Autodesk Inventor part; units mm, degrees
ref_plane "YZ Plane" through (0, 0, 0) normal (1, 0, 0) x (0, 1, 0)
ref_plane "XZ Plane" through (0, 0, 0) normal (0, 1, 0) x (-1, 0, 0)
ref_plane "XY Plane" through (0, 0, 0) normal (0, 0, 1) x (1, 0, 0)
sketch "Sketch1" plane through (0, 0, 0) normal (0, 0, 1) x (1, 0, 0)
  circle A0 centre (45.5, -15.3826) radius 3
  circle A1 centre (-45.5, -15.3826) radius 3
  line L0 (44.6636, 0.7689) -> (35.6636, 0.7689)
  line L1 (33.6636, 2.7689) -> (33.6636, 5.2689)
  line L2 (46.6636, 5.2689) -> (46.6636, 2.7689)
  line L3 (29.9455, -2.1666) -> (-2.0545, -2.1666)
  line L4 (-4.0545, -0.1666) -> (-4.0545, 2.8334)
  line L5 (31.9455, 2.8334) -> (31.9455, -0.1666)
  circle A2 centre (89.024, -15.4039) radius 1.5
  circle A3 centre (65.024, -15.4039) radius 1.5
  circle A4 centre (89.024, 8.5961) radius 1.5
  circle A5 centre (65.024, 8.5961) radius 1.5
  arc A6 (67.8322, 7.6809) -> (67.8322, -14.4886) centre (77.024, -3.4039) ccw
  line L6 (69.3366, 7.4111) -> (71.8641, 3.0334)
  arc A7 (71.8641, 3.0334) -> (71.8641, -9.8411) centre (77.024, -3.4039) ccw
  line L7 (71.8641, -9.8411) -> (69.3366, -14.2188)
  arc A8 (67.8322, -14.4886) -> (69.3366, -14.2188) centre (68.4705, -13.7188) ccw
  arc A9 (69.3366, 7.4111) -> (67.8322, 7.6809) centre (68.4705, 6.9111) ccw
  arc A10 (91.2195, -0.986) -> (72.0202, 10.0988) centre (77.024, -3.4039) ccw
  arc A11 (72.0202, 10.0988) -> (71.5016, 8.6611) centre (72.3677, 9.1611) ccw
  line L8 (74.0291, 4.2834) -> (71.5016, 8.6611)
  arc A12 (85.1787, -2.1539) -> (74.0291, 4.2834) centre (77.024, -3.4039) ccw
  line L9 (90.2337, -2.1539) -> (85.1787, -2.1539)
  arc A13 (90.2337, -2.1539) -> (91.2195, -0.986) centre (90.2337, -1.1539) ccw
  line L10 (85.1787, -4.6539) -> (90.2337, -4.6539)
  arc A14 (91.2195, -5.8218) -> (90.2337, -4.6539) centre (90.2337, -5.6539) ccw
  arc A15 (72.0202, -16.9065) -> (91.2195, -5.8218) centre (77.024, -3.4039) ccw
  arc A16 (71.5016, -15.4688) -> (72.0202, -16.9065) centre (72.3677, -15.9688) ccw
  line L11 (71.5016, -15.4688) -> (74.0291, -11.0911)
  arc A17 (74.0291, -11.0911) -> (85.1787, -4.6539) centre (77.024, -3.4039) ccw
  circle A18 centre (-64.8953, -15.374) radius 1.5
  circle A19 centre (-88.8953, -15.374) radius 1.5
  circle A20 centre (-88.8953, 8.626) radius 1.5
  circle A21 centre (-64.8953, 8.626) radius 1.5
  arc A22 (-62.6997, -0.956) -> (-81.8991, 10.1287) centre (-76.8953, -3.374) ccw
  arc A23 (-81.8991, 10.1287) -> (-82.4176, 8.691) centre (-81.5516, 9.191) ccw
  line L12 (-79.8901, 4.3133) -> (-82.4176, 8.691)
  line L13 (-84.5827, 7.441) -> (-82.0552, 3.0633)
  arc A24 (-84.5827, 7.441) -> (-86.087, 7.7108) centre (-85.4487, 6.941) ccw
  arc A25 (-86.087, 7.7108) -> (-86.087, -14.4587) centre (-76.8953, -3.374) ccw
  arc A26 (-82.0552, 3.0633) -> (-82.0552, -9.8112) centre (-76.8953, -3.374) ccw
  arc A27 (-68.7405, -2.124) -> (-79.8901, 4.3133) centre (-76.8953, -3.374) ccw
  line L14 (-63.6855, -2.124) -> (-68.7405, -2.124)
  arc A28 (-63.6855, -2.124) -> (-62.6997, -0.956) centre (-63.6855, -1.124) ccw
  line L15 (-68.7405, -4.624) -> (-63.6855, -4.624)
  arc A29 (-62.6997, -5.7919) -> (-63.6855, -4.624) centre (-63.6855, -5.624) ccw
  arc A30 (-81.8991, -16.8766) -> (-62.6997, -5.7919) centre (-76.8953, -3.374) ccw
  arc A31 (-79.8901, -11.0612) -> (-68.7405, -4.624) centre (-76.8953, -3.374) ccw
  line L16 (-82.4176, -15.4389) -> (-79.8901, -11.0612)
  arc A32 (-82.4176, -15.4389) -> (-81.8991, -16.8766) centre (-81.5516, -15.9389) ccw
  line L17 (-82.0552, -9.8112) -> (-84.5827, -14.1889)
  arc A33 (-86.087, -14.4587) -> (-84.5827, -14.1889) centre (-85.4487, -13.6889) ccw
  line L18 (-2.0545, 4.8334) -> (29.9455, 4.8334)
  line L19 (35.6636, 7.2689) -> (44.6636, 7.2689)
  arc A34 (-4.0545, -0.1666) -> (-2.0545, -2.1666) centre (-2.0545, -0.1666) ccw
  arc A35 (-2.0545, 4.8334) -> (-4.0545, 2.8334) centre (-2.0545, 2.8334) ccw
  arc A36 (31.9455, 2.8334) -> (29.9455, 4.8334) centre (29.9455, 2.8334) ccw
  arc A37 (29.9455, -2.1666) -> (31.9455, -0.1666) centre (29.9455, -0.1666) ccw
  arc A38 (33.6636, 2.7689) -> (35.6636, 0.7689) centre (35.6636, 2.7689) ccw
  arc A39 (35.6636, 7.2689) -> (33.6636, 5.2689) centre (35.6636, 5.2689) ccw
  arc A40 (46.6636, 5.2689) -> (44.6636, 7.2689) centre (44.6636, 5.2689) ccw
  arc A41 (44.6636, 0.7689) -> (46.6636, 2.7689) centre (44.6636, 2.7689) ccw
  line L20 (-87.4504, 24.6174) -> (-57.4504, 24.6174)
  line L21 (-87.4504, 19.6174) -> (-87.4504, 24.6174)
  line L22 (-87.4504, 19.6174) -> (-57.4504, 19.6174)
  line L23 (-57.4504, 19.6174) -> (-57.4504, 24.6174)
  line L24 (-27.4504, 19.6174) -> (27.5496, 19.6174)
  line L25 (27.5496, 19.6174) -> (27.5496, 24.6174)
  line L26 (-27.4504, 24.6174) -> (27.5496, 24.6174)
  line L27 (-27.4504, 19.6174) -> (-27.4504, 24.6174)
  line L28 (57.5496, 19.6174) -> (87.5496, 19.6174)
  line L29 (87.5496, 19.6174) -> (87.5496, 24.6174)
  line L30 (57.5496, 24.6174) -> (87.5496, 24.6174)
  line L31 (57.5496, 19.6174) -> (57.5496, 24.6174)
  line L32 (-98.9504, -25.3833) -> (-98.9504, -33.3826)
  line L33 (99.0496, -33.3826) -> (-98.9504, -33.3826)
  line L34 (-98.9504, 24.6174) -> (-93.9504, 24.6174)
  line L35 (-93.9504, 24.6174) -> (-93.9504, 9.6159)
  line L36 (-98.9504, 9.6159) -> (-93.9504, 9.6159)
  line L37 (-98.9504, 9.6159) -> (-98.9504, -10.3841)
  line L38 (-98.9504, -10.3841) -> (-93.9504, -10.3841)
  line L39 (-93.9504, -10.3841) -> (-93.9504, -25.3833)
  line L40 (-98.9504, -25.3833) -> (-93.9504, -25.3833)
  line L41 (99.0496, -25.3833) -> (99.0496, -33.3833)
  line L42 (94.0496, -25.3833) -> (99.0496, -25.3833)
  line L43 (94.0496, -10.3841) -> (94.0496, -25.3833)
  line L44 (94.0496, -10.3841) -> (99.0496, -10.3841)
  line L45 (99.0496, 9.6159) -> (99.0496, -10.3841)
  line L46 (94.0496, 9.6159) -> (99.0496, 9.6159)
  line L47 (94.0496, 24.6174) -> (94.0496, 9.6159)
  line L48 (94.0496, 24.6174) -> (99.0496, 24.6174)
  line L49 (-98.9504, 24.6174) -> (-98.9504, 32.6174)
  line L50 (-98.9504, 32.6174) -> (99.0496, 32.6174)
  line L51 (99.0496, 32.6174) -> (99.0496, 24.6174)
  line L52 (-22.6436, -2.2792) -> (-22.6436, -8.2792)
  line L53 (-35.6436, -0.2792) -> (-24.6436, -0.2792)
  line L54 (-24.6436, -10.2792) -> (-35.6436, -10.2792)
  line L55 (-37.6436, -8.2792) -> (-37.6436, -2.2792)
  arc A42 (-35.6436, -0.2792) -> (-37.6436, -2.2792) centre (-35.6436, -2.2792) ccw
  arc A43 (-22.6436, -2.2792) -> (-24.6436, -0.2792) centre (-24.6436, -2.2792) ccw
  arc A44 (-24.6436, -10.2792) -> (-22.6436, -8.2792) centre (-24.6436, -8.2792) ccw
  arc A45 (-37.6436, -8.2792) -> (-35.6436, -10.2792) centre (-35.6436, -8.2792) ccw
  line L56 (-5.5869, 3.8805) -> (-5.5869, -1.877)
  line L57 (-7.5869, -3.877) -> (-13.5192, -3.877)
  line L58 (-15.5192, -1.877) -> (-15.5192, 3.8805)
  line L59 (-13.5192, 5.8805) -> (-7.5869, 5.8805)
  arc A46 (-13.5192, 5.8805) -> (-15.5192, 3.8805) centre (-13.5192, 3.8805) ccw
  arc A47 (-15.5192, -1.877) -> (-13.5192, -3.877) centre (-13.5192, -1.877) ccw
  arc A48 (-5.5869, 3.8805) -> (-7.5869, 5.8805) centre (-7.5869, 3.8805) ccw
  arc A49 (-7.5869, -3.877) -> (-5.5869, -1.877) centre (-7.5869, -1.877) ccw
  point P0 (-90.9348, -30.6649)
  point P1 (27.5, 24.6174)
  point P2 (0, 0)
  point P3 (-22.6436, -0.2792)
  point P4 (-22.6436, -10.2792)
  point P5 (-37.6436, -0.2792)
  point P6 (-37.6436, -10.2792)
  point P7 (-2.0545, 2.8334)
  dimension "d22" = 91
  dimension "d27" = 7
  dimension "d28" = 36
  dimension "d29" = 13
  dimension "d30" = 6.5
  dimension "d35" = 18
  dimension "d36" = 18
  dimension "d37" = 66
  dimension "d38" = 45.5
  dimension "d39" = 6
  dimension "d40" = 6
  dimension "d41" = 198
extrude "Extrusion1" add sketch "Sketch1" along normal blind 5
sketch "Sketch2" plane through (0, 0, 5) normal (0, 0, 1) x (1, 0, 0)
  line L0 (-44.5, 11.026) -> (44.5, 11.026)
  line L1 (48.5, 7.026) -> (48.5, -6.974)
  line L2 (44.5, -10.974) -> (-44.5, -10.974)
  line L3 (-48.5, -6.974) -> (-48.5, 7.026)
  arc A0 (-44.5, 11.026) -> (-48.5, 7.026) centre (-44.5, 7.026) ccw
  arc A1 (48.5, 7.026) -> (44.5, 11.026) centre (44.5, 7.026) ccw
  arc A2 (44.5, -10.974) -> (48.5, -6.974) centre (44.5, -6.974) ccw
  arc A3 (-48.5, -6.974) -> (-44.5, -10.974) centre (-44.5, -6.974) ccw
  line L4 (99.0496, -10.3841) -> (99.0496, 9.6159)
  line L5 (-98.9504, -33.3826) -> (99.0496, -33.3826)
  circle A4 centre (-45.5, -15.3826) radius 3
  circle A5 centre (45.5, -15.3826) radius 3
  arc A6 (-62.6997, -0.956) -> (-81.8991, 10.1287) centre (-76.8953, -3.374) ccw
  point P0 (0, 0)
  point P1 (-76.8953, -3.374)
  dimension "d48" = 4
  dimension "d58" = 97
  dimension "d59" = 22
  dimension "d60" = 50.5496
  dimension "d61" = 22.4087
extrude "Extrusion2" cut sketch "Sketch2" against normal up to next contours L0 A1 L1 A2 L2 A3 L3 A0
sketch "Sketch3" plane through (0, 0, 5) normal (0, 0, 1) x (1, 0, 0)
  line L0 (-92.421, 12.1859) -> (-62.2986, 12.1859)
  line L1 (-62.2986, 12.1859) -> (-62.2986, -19.0319)
  line L2 (-62.2986, -19.0319) -> (-92.421, -19.0319)
  line L3 (-92.421, -19.0319) -> (-92.421, 12.1859)
  line L4 (-92.421, 12.1859) -> (-62.2986, -19.0319) construction
  line L5 (-62.2986, 12.1859) -> (-92.421, -19.0319) construction
  line L6 (62.2986, 11.0377) -> (92.6949, 11.0377)
  line L7 (92.6949, 11.0377) -> (92.6949, -17.8837)
  line L8 (92.6949, -17.8837) -> (62.2986, -17.8837)
  line L9 (62.2986, -17.8837) -> (62.2986, 11.0377)
  line L10 (62.2986, 11.0377) -> (92.6949, -17.8837) construction
  line L11 (92.6949, 11.0377) -> (62.2986, -17.8837) construction
  point P0 (0, 0)
  point P1 (-77.3598, -3.423)
  point P2 (77.4968, -3.423)
extrude "Extrusion3" add sketch "Sketch3" against normal blind 10
properties part number "case bottom back" material "Titanium"
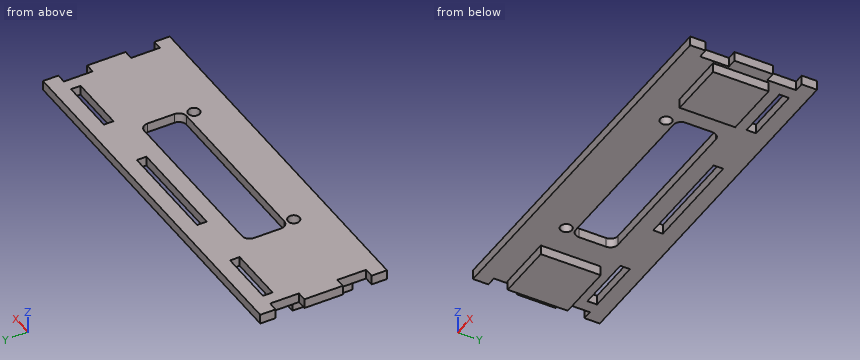
The model under review builds one solid part; all positions refer to its coordinate system, in mm. Round coordinates to 2 decimals unless told otherwise and drop trailing zeros. Order: outer loops, then holes, each group sorted by start corner. A loop starts at its lowest first (then second) coordinate and runs counter-clockwise, first axis right, second up. Notation, with made-up numbers: (-28.5, 17) -> (-23.5, 17) arc R29 ccw to (-23.5, 43) -> close; hole circle Ø6 at (84, -36.5). An arc over 180 degrees is marked (long way). Use a Markdown table: item, result.
Q1. We need section C-C on x = -60. Write out the cut boundary in (y, z), then the cut area to 3 significant figures.
Values:
| item | result |
|---|---|
| outline | (-33.38, 0) -> (19.62, 0) -> (19.62, 5) -> (-33.38, 5) -> close; (24.62, 0) -> (32.62, 0) -> (32.62, 5) -> (24.62, 5) -> close |
| area | 305 mm^2 |
Q2. For line 1 (Y direction, x = -59.5, z = 3); line 2 (X direction, y = 2, z = 0.75); line 3 (Y direction, x = -25.5, z = 1.5), list the stretches that pass through material, from the lowest coordinate up.
Values:
| item | result |
|---|---|
| line 1 | y = -33.38 to 19.62, 24.62 to 32.62 |
| line 2 | x = -98.95 to -48.5, 48.5 to 99.05 |
| line 3 | y = -33.38 to -10.97, 11.03 to 19.62, 24.62 to 32.62 |
Q3. We need section D-D on y = -21. Write out the cut boundary in (x, z).
Values:
| item | result |
|---|---|
| outline | (-93.95, 0) -> (94.05, 0) -> (94.05, 5) -> (-93.95, 5) -> close |
Q4. We need section A-A on x = -21. Write out the cut boundary in (y, z), then the cut area to 3 significant figures.
Values:
| item | result |
|---|---|
| outline | (-33.38, 0) -> (-10.97, 0) -> (-10.97, 5) -> (-33.38, 5) -> close; (11.03, 0) -> (19.62, 0) -> (19.62, 5) -> (11.03, 5) -> close; (24.62, 0) -> (32.62, 0) -> (32.62, 5) -> (24.62, 5) -> close |
| area | 195 mm^2 |
Q5. Clearance check with flat-ended pins moving along their axes: P1, Ø6, axis at x = -22, z = -4, coming from the +Y side; P2, Ø2.5, axis at y = -6, z = -2, coming from the +X side; P3, Ø1, axis at y = -6.5, z = -3, coming from the -X side; P4, Ø1.5, axis at y = 23, z = 2.5, coming from the -X side. State where each tip first meets the part, or that it passes through.
Values:
| item | result |
|---|---|
| P1 | passes through |
| P2 | stops at x = 92.69 |
| P3 | stops at x = -92.42 |
| P4 | stops at x = -93.95 |
Q6. We need section B-B on z = -2. Write out the cut boundary in (x, y).
Values:
| item | result |
|---|---|
| outline | (-92.42, -19.03) -> (-62.3, -19.03) -> (-62.3, 12.19) -> (-92.42, 12.19) -> close; (62.3, -17.88) -> (92.69, -17.88) -> (92.69, 11.04) -> (62.3, 11.04) -> close |
